The model under review builds one solid part; all positions refer to its coordinate system, in mm. A direction names the side the tool comes from. Give positions to 0.01 mm unless a question says otherwise; leave off trailing zeros. Loops run counter-clockwise (first coordinate to the right, second up) from the corner with the lowest first, then second, coordinate; pieces in that order, holes last. Notation, with made-up numbers: M 25.25,21 L 64.25,21 A34 ccw 64.25,53 Z; hole C -17.5,38 d3. An arc over 180 degrees is marked long. Put each result on its own line as item: value. Start each with the question number.
```python
from build123d import *

# Parameters (mm, degrees)
F1_DEPTH = 76.2
F2_R     = 5.08
F3_R     = 5.08


with BuildPart() as f1:
    # F0 (on Front) → F1 (new body)
    with BuildSketch(Plane.XZ):
        Polygon((-552.45, 0), (0, 0), (0, 38.1), (-6.35, 38.1), (-6.35, 6.35), (-546.1, 6.35), (-546.1, 38.1), (-552.45, 38.1), (-552.45, 6.35), align=None)
    extrude(amount=F1_DEPTH)

    # F2
    f2_edges = [f1.edges().sort_by_distance(p)[0] for p in [
        (-552.45, -38.1, 0),
    ]]
    fillet(f2_edges, radius=F2_R)

    # F3
    f3_edges = [f1.edges().sort_by_distance(p)[0] for p in [
        (0, -38.1, 0),
    ]]
    fillet(f3_edges, radius=F3_R)


solid = f1.part
```
Item 1: Consider section A-A, the plane z = 21. Write out the cut boundary in (x, y), plus the area to 3 significant figures.
Item 2: Consider section B-B, the plane y = -7.5. Write out the cut boundary in (x, z).
Item 3: Clearance check with flat-ended pins moving along their axes: pin 1 Ø1 at (x, y) = (-65, -13.5) entering from +Z; pin 2 Ø12 at (x, z) = (-188, 14.5) entering from +Y. State where each tip first meets the part, or that it passes through.
Item 4: To check wall thickness, follow L1, parallel to X at y = -24.5, z = 8.5; L2, parallel to Z at x = -515.5, y = -51; L3, parallel to X at y = -38.5, z = 3.5. State the ranges of each line that lie inside material, in increasing order. Write a range as [from, to].
Item 5: Draft analysis for pull direction X (two halves, no side actions). For faces 1 (the flat face through (-6.35, -38, 22)), 2 (the flat face through (-278, -76.2, 4)), 3 (the flat face through (-552.45, -38, 22)), state which applies: +X half, -X half, draft (parallel to the pull), parting line (faces both ways), or undercut.
Item 6: Consider section C-C, the plane x = -57.5. Write out the cut boundary in (y, z), plus the area to 3 significant figures.
Item 7: Tool access review of faces 4 (the flat face through (-278, 0, 4)), 5 (the flat face through (-272, -38, 6.35)): name each direction out of +Z, -Z, +X, -X, +Y, -Y from which nothing blocks a thin tool from reaching the whole face with its end or side.
Report:
1. outline: M -552.45,-76.2 L -546.1,-76.2 L -546.1,0 L -552.45,0 Z; M -6.35,-76.2 L 0,-76.2 L 0,0 L -6.35,0 Z
1. area: 968 mm²
2. outline: M -552.45,5.08 A5.08 ccw -547.37,0 L -5.08,0 A5.08 ccw 0,5.08 L 0,38.1 L -6.35,38.1 L -6.35,6.35 L -546.1,6.35 L -546.1,38.1 L -552.45,38.1 Z
3. pin 1: z = 6.35
3. pin 2: through
4. L1: [-552.45, -546.1], [-6.35, 0]
4. L2: [0, 6.35]
4. L3: [-552.2, -0.25]
5. face 1: undercut
5. face 2: draft
5. face 3: -X half
6. outline: M -76.2,0 L 0,0 L 0,6.35 L -76.2,6.35 Z
6. area: 484 mm²
7. face 4: +Z, -Z, +X, -X, +Y
7. face 5: +Z, +Y, -Y
